Part print with two shaded views. Sizes in mm from the minimum x, y, z corner. Coordinates: 2 decimals unless noted, no trailing zeros. Order: outer loops, then holes, each group sorted by start corner. A loop starts at its lowest first (then second) coordinate and runs counter-clockwise, first axis right, second up. Notation, with made-up numbers: (-14.75, -10) - (37.25, -10) arc R25 cw to (37.25, 14) - close; hole circle Ø10 at (54, -30). An arc over 180 degrees is marked (long way). Return JSON: item names as keys, results as strings.
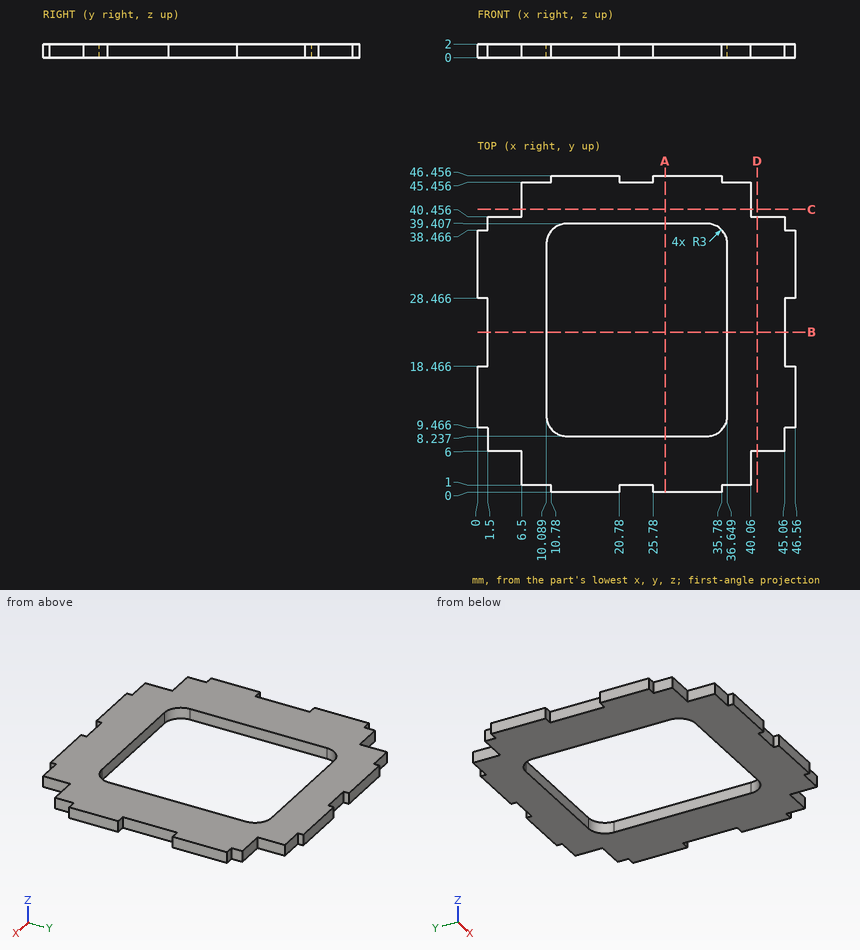
Item 1: Band-saw the part on D-D, the plane x = 41. List the corners of the cut face in (y, z).
Findings below:
{"outline": "(6, 0) - (40.46, 0) - (40.46, 2) - (6, 2) - close"}
Item 2: Band-saw the part on A-A, the plane x = 27.5. List the corners of the cut face in (y, z).
Findings below:
{"outline": "(0, 0) - (8.24, 0) - (8.24, 2) - (0, 2) - close; (39.41, 0) - (46.46, 0) - (46.46, 2) - (39.41, 2) - close"}
Item 3: Wall check: L1, parallel to Y at x = 22, z = 1.5; L2, parallel to Y at x = 15, z = 1.3; L3, parallel to X at y = 31.5, z = 1.4. Give the ranges that are in metal, low to high. Write a range as [from, to].
Findings below:
{"L1": "y = [1, 8.24], [39.41, 45.46]", "L2": "y = [0, 8.24], [39.41, 46.46]", "L3": "x = [0, 10.09], [36.65, 46.56]"}
Item 4: Band-saw the part on C-C, the plane y = 41.5. List the corners of the cut face in (x, z).
Findings below:
{"outline": "(6.5, 0) - (40.06, 0) - (40.06, 2) - (6.5, 2) - close"}
Item 5: Drop flat-ended pins along their axis: P1, Ø0.5, axis at y = 46, z = 0.5, coming from the +X side; P2, Ø1.1, axis at y = 0.5, z = 0.5, coming from the +X side; P3, Ø0.5, axis at y = 0.5, z = 1, coming from the -X side. Give the stop position or say it passes through.
Findings below:
{"P1": "stops at x = 35.78", "P2": "stops at x = 40.06", "P3": "stops at x = 10.78"}
Item 6: Band-saw the part on B-B, the plane y = 23.5. List the corners of the cut face in (x, z), then the cut area to 3 significant figures.
Findings below:
{"outline": "(1.5, 0) - (10.09, 0) - (10.09, 2) - (1.5, 2) - close; (36.65, 0) - (45.06, 0) - (45.06, 2) - (36.65, 2) - close", "area": "34.0 mm²"}
